Could you check a few things on this model? Use its own coordinates, in mm. Face numbers are marked on the shaded views. Coordinates: 2 decimals unless noted, no trailing zeros. Loops run counter-clockwise (first coordinate to the right, second up) from the corner with the lowest first, then second, coordinate; pieces in that order, holes last. Notation, with made-up numbers: (31.25, 59) -> (40.25, 59) arc R33 ccw to (40.25, 93) -> close; hole circle Ø6 at (-33.75, 73). An arc over 180 degrees is marked (long way). One line per question, with ' | ' between items. Start each with the question number.
(1) Suppose I cut it at A-A (z = 45.99). Please give me the cut outline in (x, y), plus the area to 3 significant figures.
(2) If I drill on line 1 along Z through (x, y) = (-3.5, 10.75); line 2 along Z through (x, y) = (-2.25, 9) (3 decimals); line 3 along X through (y, z) = (15, -45.99), over which ranges is the centre line in solid material (lowest first)?
(3) Suppose I cut it at B-B (y = 17.25). Please give me the cut outline in (x, z).
(4) If we mould it in two halves opening along Z, with no side actions, what happens to the marked faces 1 and 2? For each: pulls with the +Z half, pulls with the -Z half, needs draft (parallel to the pull), parting line crosses it, or undercut.
(5) Suppose I cut it at C-C (z = -31). Please give me the cut outline in (x, y).
(6) I'm going to push flat-ended pins straight in: pin 1 Ø4 at (x, z) = (-1, 6.5) entering from -Y; pin 2 Ø1.9 at (x, z) = (-1.016, 45.99) entering from -Y. Where does each tip first touch, or does it pass through?
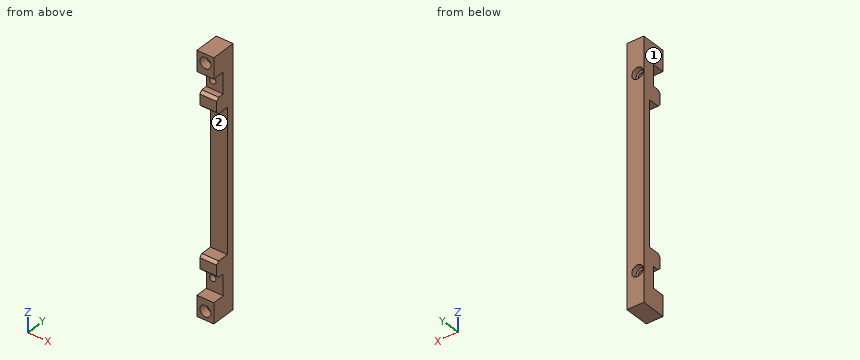
```python
from build123d import *

# Parameters (mm, degrees)
SKETCH1_W                        = 8.128
SKETCH1_H                        = 127
BOSS_EXTRUDE1_DEPTH              = 18.288
SKETCH2_W                        = 8.128
SKETCH2_H                        = 104.14
CUT_EXTRUDE1_DEPTH               = 8.128
SKETCH4_W                        = 8.128
SKETCH4_H                        = 10.16
CUT_EXTRUDE2_DEPTH               = 4.064
SKETCH5_W                        = 8.128
SKETCH5_H                        = 34.29
CUT_EXTRUDE4_DEPTH               = 6.604
CBORE_FOR_M2_5_SHCS1_D           = 3.1
CBORE_FOR_M2_5_SHCS1_CBORE_D     = 5.5
CBORE_FOR_M2_5_SHCS1_CBORE_DEPTH = 2.5
CHAMFER1_SIZE                    = 1.27
SKETCH17_W                       = 8.128
SKETCH17_H                       = 127
CUT_EXTRUDE5_DEPTH               = 6.35
SKETCH18_W                       = 8.128
SKETCH18_H                       = 1.546440773
CUT_EXTRUDE6_DEPTH               = 12.938
SKETCH19_W                       = 8.128
SKETCH19_H                       = 1.507728281
CUT_EXTRUDE7_DEPTH               = 12.938


with BuildPart() as part:
    # Sketch1 → Boss-Extrude1 (new body)
    with BuildSketch(Plane(origin=(0, 0, 0), x_dir=(1, 0, 0), z_dir=(0, 1, 0))):
        Rectangle(SKETCH1_W, SKETCH1_H)
    extrude(amount=BOSS_EXTRUDE1_DEPTH)

    # Sketch2 → Cut-Extrude1 (cut)
    with BuildSketch(Plane.XZ):
        Rectangle(SKETCH2_W, SKETCH2_H)
    extrude(amount=-CUT_EXTRUDE1_DEPTH, mode=Mode.SUBTRACT)

    # Sketch4 → Cut-Extrude2 (cut)
    with BuildSketch(Plane.XZ.offset(-8.128)):
        with Locations((0, -46.99)):
            Rectangle(SKETCH4_W, SKETCH4_H)
    cut_extrude2 = extrude(amount=-CUT_EXTRUDE2_DEPTH, mode=Mode.SUBTRACT)

    # Sketch5 → Cut-Extrude4 (cut)
    with BuildSketch(Plane.XZ.offset(-8.128)):
        with Locations((0, -17.145)):
            Rectangle(SKETCH5_W, SKETCH5_H)
    cut_extrude4 = extrude(amount=-CUT_EXTRUDE4_DEPTH, mode=Mode.SUBTRACT)

    # CBORE for M2.5 SHCS1 (through all)
    with Locations(Plane(origin=(0, 18.288, 0), x_dir=(1, 0, 0), z_dir=(0, 1, 0))):
        with Locations((-1.016, 45.99)):
            cbore_for_m2_5_shcs1 = CounterBoreHole(CBORE_FOR_M2_5_SHCS1_D / 2, CBORE_FOR_M2_5_SHCS1_CBORE_D / 2, CBORE_FOR_M2_5_SHCS1_CBORE_DEPTH)

    # Mirror1: Cut-Extrude2, Cut-Extrude4 across plane
    add(cut_extrude2.mirror(Plane(origin=(4.064, 14.732, 0), x_dir=(1, 0, 0), z_dir=(0, 0, 1))), mode=Mode.SUBTRACT)
    add(cut_extrude4.mirror(Plane(origin=(4.064, 14.732, 0), x_dir=(1, 0, 0), z_dir=(0, 0, 1))), mode=Mode.SUBTRACT)

    # Mirror2: CBORE for M2.5 SHCS1 across plane
    add(cbore_for_m2_5_shcs1.mirror(Plane.XY), mode=Mode.SUBTRACT)

    # Sketch15 → Ø1.0mm Dowel Hole1 (revolve, cut)
    with BuildSketch(Plane(origin=(0, 0, -57.785), x_dir=(0, 0, -1), z_dir=(1, 0, 0))):
        Polygon((0, 0), (0, 11.94227264), (2.65, 10.349992), (2.65, 0), align=None)
    f_1_0mm_dowel_hole1 = revolve(axis=Axis((0, -6.35, -57.785), (0, 1, 0)), mode=Mode.SUBTRACT)

    # Mirror3: Ø1.0mm Dowel Hole1 across plane
    add(f_1_0mm_dowel_hole1.mirror(Plane.XY), mode=Mode.SUBTRACT)

    # Chamfer1
    chamfer1_edges = [part.edges().sort_by_distance(p)[0] for p in [
        (0, 0, 52.07),
        (0, 0, -52.07),
        (0, 8.128, -41.91),
        (0, 0, 63.5),
        (0, 8.128, -34.29),
        (0, 0, -63.5),
        (0, 8.128, 41.91),
        (0, 8.128, 34.29),
    ]]
    chamfer(chamfer1_edges, length=CHAMFER1_SIZE)

    # Sketch17 → Cut-Extrude5 (cut)
    with BuildSketch(Plane.XZ):
        Rectangle(SKETCH17_W, SKETCH17_H)
    extrude(amount=-CUT_EXTRUDE5_DEPTH, mode=Mode.SUBTRACT)

    # Sketch18 → Cut-Extrude6 (cut, through all)
    with BuildSketch(Plane.XZ.offset(-6.35)):
        with Locations((0, -62.726779614)):
            Rectangle(SKETCH18_W, SKETCH18_H)
    extrude(amount=-CUT_EXTRUDE6_DEPTH, mode=Mode.SUBTRACT)

    # Sketch19 → Cut-Extrude7 (cut, through all)
    with BuildSketch(Plane.XZ.offset(-6.35)):
        with Locations((0, 62.74613586)):
            Rectangle(SKETCH19_W, SKETCH19_H)
    extrude(amount=-CUT_EXTRUDE7_DEPTH, mode=Mode.SUBTRACT)


solid = part.part
```
Checks:
1) outline: (-4.06, 12.19) -> (-2.57, 12.19) -> (-2.57, 15.79) -> (-3.77, 15.79) -> (-3.77, 18.29) -> (-4.06, 18.29) -> close; (0.53, 12.19) -> (4.06, 12.19) -> (4.06, 18.29) -> (1.73, 18.29) -> (1.73, 15.79) -> (0.53, 15.79) -> close | area: 24.7 mm^2
2) line 1: z = -61.95 to -52.07, -41.91 to -34.29, 34.29 to 41.91, 52.07 to 61.99 | line 2: z = -61.954 to -59.185, -56.385 to -52.07, -41.512 to -34.688, 34.688 to 41.512, 52.07 to 56.385, 59.185 to 61.992 | line 3: x = -4.06 to -2.57, 0.53 to 4.06
3) outline: (-4.06, -61.95) -> (4.06, -61.95) -> (4.06, 61.99) -> (-4.06, 61.99) -> close; hole circle Ø5.5 at (-1.02, -45.99); hole circle Ø5.5 at (-1.02, 45.99)
4) face 1: needs draft | face 2: undercut
5) outline: (-4.06, 14.73) -> (4.06, 14.73) -> (4.06, 18.29) -> (-4.06, 18.29) -> close
6) pin 1: stops at y = 14.73 | pin 2: passes through
